from build123d import *

# Parameters (mm, degrees)
F1_DEPTH = 120
F2_W     = 35.058874
F2_H     = 4.015654
F3_DEPTH = 5
F4_W     = 5
F4_H     = 4.015654
F5_DEPTH = 25
F6_W     = 5
F6_H     = 4.015654
F7_DEPTH = 25


with BuildPart() as f1:
    # F0 (on Top) → F1 (new body)
    with BuildSketch(Plane.XY):
        Polygon((-13.854021, -31.714595), (-18.824584, -43.714595), (26.175416, -43.714595), (21.204853, -31.714595), align=None)
    extrude(amount=F1_DEPTH)

    # F2 (on face) → F3 (cut)
    with BuildSketch(Plane(origin=(0, -31.714595, 0), x_dir=(-1, 0, 0), z_dir=(0, 1, 0))):
        with Locations((-3.675416, 14.314208)):
            Rectangle(F2_W, F2_H)
    extrude(amount=-F3_DEPTH, mode=Mode.SUBTRACT)

    # F4 (on face) → F5 (cut)
    with BuildSketch(Plane.YZ.offset(-13.854021)):
        with Locations((-34.214595, 14.314208)):
            Rectangle(F4_W, F4_H)
    extrude(amount=-F5_DEPTH, mode=Mode.SUBTRACT)

    # F6 (on face) → F7 (cut)
    with BuildSketch(Plane(origin=(21.204853, 0, 0), x_dir=(0, -1, 0), z_dir=(-1, 0, 0))):
        with Locations((34.214595, 14.314208)):
            Rectangle(F6_W, F6_H)
    extrude(amount=-F7_DEPTH, mode=Mode.SUBTRACT)


solid = f1.part
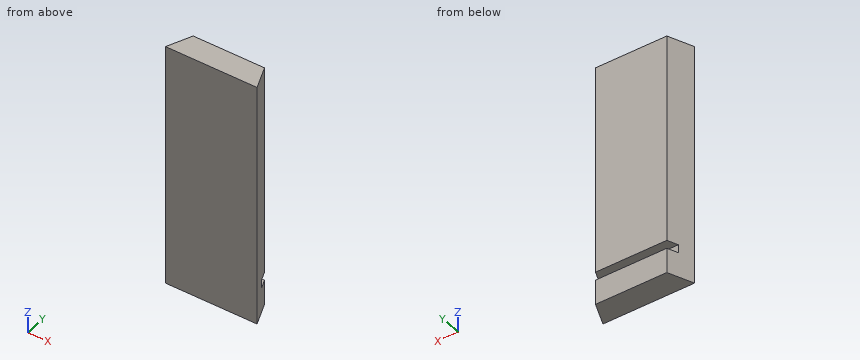
Could you check a few things on this model? Use its own coordinates, in mm. Give positions to 0.01 mm unless a question says otherwise; leave off trailing zeros. Loops run counter-clockwise (first coordinate to the right, second up) from the corner with the lowest first, then second, coordinate; pieces in that order, holes last. Notation, with made-up numbers: (41, 66) -> (94, 66) arc R25 ccw to (94, 90) -> close; hole circle Ø4 at (-35, 26). An arc over 180 degrees is marked (long way). Answer as CSV lines item,"result". Start each with the question number.
(1) If we section it at A-A on y = -35.25: Write out the boundary of the cut face in (x, z).
(2) If we section it at B-B on z = 51.5: Write out the boundary of the cut face in (x, y).
(3) I need wall thicknesses on probe 1 along Z at (x, y) = (-14, -36); probe 2 along Y at (x, z) = (3.5, 14); probe 3 along X at (y, z) = (-36.75, 21). Which ranges of each line are inside material? Lowest first, please.
(4) If we section it at C-C on y = -41.25: Write out the boundary of the cut face in (x, z).
(5) I'm going to push flat-ended pins straight in: pin 1 Ø1 at (y, z) = (-33, 16) entering from +X; pin 2 Ø1.2 at (x, z) = (1.5, 14) entering from +Y; pin 3 Ø4 at (y, z) = (-40.5, 73.5) entering from +X. Where does each tip first touch, or does it pass through?
Computed:
1,outline,"(-15.32, 0) -> (22.67, 0) -> (22.67, 12.31) -> (-15.32, 12.31) -> close; (-15.32, 16.32) -> (22.67, 16.32) -> (22.67, 120) -> (-15.32, 120) -> close"
2,outline,"(-18.82, -43.71) -> (26.18, -43.71) -> (21.2, -31.71) -> (-13.85, -31.71) -> close"
3,probe 1,"z = 0 to 12.31, 16.32 to 120"
3,probe 2,"y = -43.71 to -36.71"
3,probe 3,"x = -15.94 to 23.29"
4,outline,"(-17.8, 0) -> (25.15, 0) -> (25.15, 120) -> (-17.8, 120) -> close"
5,pin 1,"stops at x = 21.9"
5,pin 2,"stops at y = -36.71"
5,pin 3,"stops at x = 25.67"
